```python
from build123d import *

# Parameters (mm, degrees)
SKETCH1_R           = 50
BOSS_EXTRUDE1_DEPTH = 300
SKETCH3_R           = 50
SKETCH4_R           = 50
BOSS_EXTRUDE2_DEPTH = 20
SKETCH5_R           = 20
CUT_EXTRUDE1_DEPTH  = 20
SKETCH9_R           = 20
CUT_EXTRUDE2_DEPTH  = 20


with BuildPart() as part:
    # Sketch1 → Boss-Extrude1 (new body)
    with BuildSketch(Plane(origin=(0, 0, 0), x_dir=(1, 0, 0), z_dir=(0, 1, 0))):
        with Locations(Location((0, 0, 0), (0, 0, 270))):
            Circle(SKETCH1_R)
    extrude(amount=BOSS_EXTRUDE1_DEPTH)

    # Sweep1: sweep along a path in Sketch2
    with BuildLine(Plane(origin=(0, 0, 0), x_dir=(0, 0, -1), z_dir=(1, 0, 0))) as sweep1_path:
        ThreePointArc((0, 300), (-14.644660941, 335.355339059), (-50, 350))
    # Sketch3 → Sweep1 (sweep)
    with BuildSketch(Plane(origin=(0, 300, 0), x_dir=(1, 0, 0), z_dir=(0, 1, 0))):
        Circle(SKETCH3_R)
    sweep(path=sweep1_path.line)

    # Sketch4 → Boss-Extrude2 (add)
    with BuildSketch(Plane.XY.offset(50)):
        with Locations(Location((0, 350, 0), (0, 0, 270))):
            Circle(SKETCH4_R)
    extrude(amount=BOSS_EXTRUDE2_DEPTH)

    # Sketch5 → Cut-Extrude1 (cut)
    with BuildSketch(Plane.XY.offset(70)):
        with Locations((0, 350)):
            Circle(SKETCH5_R)
    extrude(amount=-CUT_EXTRUDE1_DEPTH, mode=Mode.SUBTRACT)

    # Sketch9 → Cut-Extrude2 (cut)
    with BuildSketch(Plane.XZ):
        with Locations(Location((0, 0, 0), (0, 0, 270))):
            Circle(SKETCH9_R)
    extrude(amount=-CUT_EXTRUDE2_DEPTH, mode=Mode.SUBTRACT)


solid = part.part
```
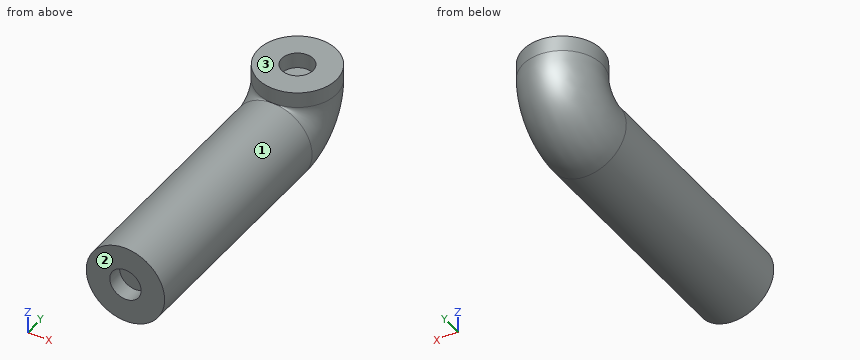
Check sheet for the modelled part. Datum: model origin and axes. Units: mm. Face numbers are marked on the shaded views. Give positions to 0.01 mm unless a question says otherwise; leave off trailing zeros. Order: outer loops, then holes, each group sorted by start corner. A loop starts at its lowest first (then second) coordinate and runs counter-clockwise, first axis right, second up. Notation, with made-up numbers: M 63,56 L 120,56 A22 ccw 120,92 Z; hole C -7.75,1.25 d7. An arc over 180 degrees is marked long. Answer in a Markdown table with one row per item.
1) Gauge pin test, flat ends, axial feed: P1, Ø12, axis at y = 313.5, z = 49, coming from the +X side; P2, Ø1, axis at x = 0, y = 270, coming from the +Z side; P3, Ø1, axis at x = 6, y = 324.5, coming from the -Z side. Record the tip position at first contact, or that the pin passes through.
Filled sheet:
| item | result |
|---|---|
| P1 | stops at x = 39.65 |
| P2 | stops at z = 50 |
| P3 | stops at z = -46.72 |
2) Thickness scan on L1, parallel to Y at x = 0, z = 60.5; L2, parallel to X at y = 11, z = 0; L3, parallel to Z at x = 1, y = 223. Record the ranges inside material, lowest first. Write a range as [from, to].
Filled sheet:
| item | result |
|---|---|
| L1 | y = [300, 330], [370, 400] |
| L2 | x = [-50, -20], [20, 50] |
| L3 | z = [-49.99, 49.99] |
3) Cross-section at A-A, the plane x = -11.5. Enter the section's corners in (y, z), plus the area to 3 significant figures.
Filled sheet:
| item | result |
|---|---|
| outline | M 0,-48.66 L 300,-48.66 A98.66 ccw 398.66,50 L 398.66,70 L 366.36,70 L 366.36,50 L 333.64,50 L 333.64,70 L 301.34,70 L 301.34,50 A1.34 cw 300,48.66 L 0,48.66 L 0,16.36 L 20,16.36 L 20,-16.36 L 0,-16.36 Z |
| area | 37,500 mm2 |
4) Cross-section at B-B, the plane y = 111.5. Enter the section's corners in (x, z).
Filled sheet:
| item | result |
|---|---|
| outline | C 0,0 d100 |
5) Cross-section at D-D, the plane x = 32. Enter the section's corners in (y, z).
Filled sheet:
| item | result |
|---|---|
| outline | M 0,-38.42 L 300,-38.42 A88.42 ccw 388.42,50 L 388.42,70 L 311.58,70 L 311.58,50 A11.58 cw 300,38.42 L 0,38.42 Z |
6) Release check for a two-part mould opening along Z. For the marked faces 1, 2 and 3 record: +Z half, -Z half, draft (parallel to the pull), parting line (faces both ways), or undercut.
Filled sheet:
| item | result |
|---|---|
| face 1 | parting line |
| face 2 | draft |
| face 3 | +Z half |
7) Cross-section at C-C, the plane x = 7. Enter the section's corners in (y, z) (3 decimals), plus the area to 3 significant figures.
Filled sheet:
| item | result |
|---|---|
| outline | M 0,-49.508 L 300,-49.508 A99.508 ccw 399.508,50 L 399.508,70 L 368.735,70 L 368.735,50 L 331.265,50 L 331.265,70 L 300.492,70 L 300.492,50 A0.492 cw 300,49.508 L 0,49.508 L 0,18.735 L 20,18.735 L 20,-18.735 L 0,-18.735 Z |
| area | 38,000 mm2 |
